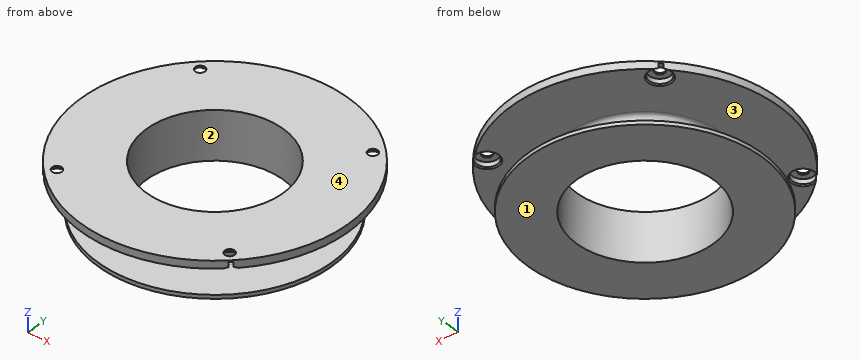
```python
from build123d import *

# Parameters (mm, degrees)
CBORE_FOR_10_BINDING_HEAD_MACHINE_S_2_COUNT = 2
CBORE_FOR_10_BINDING_HEAD_MACHINE_S_2_PITCH = 91.44
CBORE_FOR_10_BINDING_HEAD_MACHINE_S_3_COUNT = 2
CBORE_FOR_10_BINDING_HEAD_MACHINE_S_3_PITCH = 129.315688143
CBORE_FOR_10_BINDING_HEAD_MACHINE_S_4_COUNT = 2
CBORE_FOR_10_BINDING_HEAD_MACHINE_S_4_PITCH = 91.44


with BuildPart() as part:
    # Sketch1 → Revolve1 (revolve)
    with BuildSketch(Plane(origin=(0, 0, 0), x_dir=(1, 0, 0), z_dir=(0, 1, 0)), mode=Mode.PRIVATE) as revolve1_sk:
        with BuildLine():
            Line((-1.000000064, -24.96), (-1.000000064, -10.640000064))
            ThreePointArc((-1.000000064, -10.640000064), (-1.74394884, -8.84394884), (-3.540000064, -8.100000064))
            Line((-3.540000064, -8.100000064), (-24.4, -8.100000064))
            Line((-24.4, -8.100000064), (-24.4, -6.100000064))
            Line((-24.4, -6.100000064), (-1, -6.100000064))
            Line((-1, -6.100000064), (1, -6.100000064))
            Line((1, -6.100000064), (1, -31.500000128))
            Line((1, -31.500000128), (-33.29, -31.500000128))
            Line((-33.29, -31.500000128), (-33.29, -27.5))
            Line((-33.29, -27.5), (-3.540000064, -27.5))
            ThreePointArc((-3.540000064, -27.5), (-1.74394884, -26.756051224), (-1.000000064, -24.96))
        make_face()
    revolve(revolve1_sk.sketch.rotate(Axis((36.83, 0, 32.45), (0, 0, -1)), 180), axis=Axis((36.83, 0, 32.45), (0, 0, -1)))

    # Sketch7 → CBORE for #10 Binding Head Machine Screw1 (revolve, cut)
    with BuildSketch(Plane(origin=(82.55, 45.72, 27.5), x_dir=(0, 1, 0), z_dir=(1, 0, 0))):
        Polygon((0, 0), (0, 4.000000128), (2.5527, 4.000000128), (2.5527, 3.1242), (5.55625, 3.1242), (5.55625, 0.635), (6.19125, 0), align=None)
    cbore_for_10_binding_head_machine_screw = revolve(axis=Axis((82.55, 45.72, 21.15), (0, 0, 1)), mode=Mode.SUBTRACT)

    # CBORE for _10 Binding Head Machine S 2: CBORE for #10 Binding Head Machine Screw1 ×2
    with Locations(*[(-i * CBORE_FOR_10_BINDING_HEAD_MACHINE_S_2_PITCH, 0, 0) for i in range(1, CBORE_FOR_10_BINDING_HEAD_MACHINE_S_2_COUNT)]):
        add(cbore_for_10_binding_head_machine_screw, mode=Mode.SUBTRACT)

    # CBORE for _10 Binding Head Machine S 3: CBORE for #10 Binding Head Machine Screw1 ×2
    with Locations(*[Vector(-0.7071067811865476, -0.7071067811865476, 0) * (i * CBORE_FOR_10_BINDING_HEAD_MACHINE_S_3_PITCH) for i in range(1, CBORE_FOR_10_BINDING_HEAD_MACHINE_S_3_COUNT)]):
        add(cbore_for_10_binding_head_machine_screw, mode=Mode.SUBTRACT)

    # CBORE for _10 Binding Head Machine S 4: CBORE for #10 Binding Head Machine Screw1 ×2
    with Locations(*[(0, -i * CBORE_FOR_10_BINDING_HEAD_MACHINE_S_4_PITCH, 0) for i in range(1, CBORE_FOR_10_BINDING_HEAD_MACHINE_S_4_COUNT)]):
        add(cbore_for_10_binding_head_machine_screw, mode=Mode.SUBTRACT)


solid = part.part
```
Could you check a few things on this model? Use its own coordinates, in mm. Face numbers are marked on the shaded views. A direction names the side the tool comes from. Coordinates: 2 decimals unless noted, no trailing zeros. Write each loop counter-clockwise with the first axis right and the second up, starting at its lowest first coordinate (ties: lowest second). Pieces come first, ordered by that corner, then holes. Notation, with made-up numbers: (-8.5, 34.25) -> (49.5, 34.25) arc R30 ccw to (49.5, 60.25) -> close; hole circle Ø3 at (89, 45). An arc over 180 degrees is marked (long way). Return JSON: item names as keys, results as strings.
(1) Imagine slicing it at D-D, the plane z = 22. Please give me the cut outline in (x, y).
Numbers:
{"outline": "circle Ø75.66 at (36.83, 0); hole circle Ø71.66 at (36.83, 0)"}
(2) Imagine slicing it at A-A, the plane y = 0. Please give me the cut outline in (x, z).
Numbers:
{"outline": "(-33.29, 27.5) -> (-3.54, 27.5) arc R2.54 cw to (-1, 24.96) -> (-1, 10.64) arc R2.54 cw to (-3.54, 8.1) -> (-24.4, 8.1) -> (-24.4, 6.1) -> (1, 6.1) -> (1, 31.5) -> (-33.29, 31.5) -> close; (72.66, 6.1) -> (98.06, 6.1) -> (98.06, 8.1) -> (77.2, 8.1) arc R2.54 cw to (74.66, 10.64) -> (74.66, 24.96) arc R2.54 cw to (77.2, 27.5) -> (106.95, 27.5) -> (106.95, 31.5) -> (72.66, 31.5) -> close"}
(3) I'm going to push flat-ended pins straight in: pin 1 (1.5 mm diameter, centred on y = 12, z = 15, fed in from -X); pin 2 (4 mm diameter, centred on x = 38, z = 24.5, fed in from +Y); pin 3 (8 mm diameter, centred on x = 40, z = 13.5, fed in from -Y). Where does each tip first touch, or does it pass through?
Numbers:
{"pin 1": "stops at x = 0.71", "pin 2": "stops at y = 38.33", "pin 3": "stops at y = -37.99"}
(4) Imagine slicing it at B-B, the plane x = 36.83. Please give me the cut outline in (y, z), then the cut area to 3 significant figures.
Numbers:
{"outline": "(-70.12, 27.5) -> (-40.37, 27.5) arc R2.54 cw to (-37.83, 24.96) -> (-37.83, 10.64) arc R2.54 cw to (-40.37, 8.1) -> (-61.23, 8.1) -> (-61.23, 6.1) -> (-35.83, 6.1) -> (-35.83, 31.5) -> (-70.12, 31.5) -> close; (35.83, 6.1) -> (61.23, 6.1) -> (61.23, 8.1) -> (40.37, 8.1) arc R2.54 cw to (37.83, 10.64) -> (37.83, 24.96) arc R2.54 cw to (40.37, 27.5) -> (70.12, 27.5) -> (70.12, 31.5) -> (35.83, 31.5) -> close", "area": "459 mm2"}
(5) We'd pull the mould along Y, two halves only. Please class the marked faces 1 and 2: +Y half, -Y half, draft (parallel to the pull), parting line (faces both ways), or undercut.
Numbers:
{"face 1": "draft", "face 2": "undercut"}
(6) Which directions (+Z, -Z, +X, -X, +Y, -Y) give clear straight access to the entire face, cutting with the end or side of a thin tool? Please do the marked faces 3 and 4.
Numbers:
{"face 3": "none", "face 4": "+Z, +X, -X, +Y, -Y"}
(7) I need wall thicknesses on L1, parallel to Z at x = 96, y = 13; L2, parallel to Y at x = -8.89, z = 30; L3, parallel to X at y = 46, z = 29.75. Which ranges of each line are inside material? Lowest first, please.
Numbers:
{"L1": "z = 6.1 to 8.1, 27.5 to 31.5", "L2": "y = -53.16 to -51.28, -40.16 to 40.16, 51.28 to 53.16", "L3": "x = -16.09 to -14.44, -3.34 to 77, 88.1 to 89.75"}
(8) Imagine slicing it at C-C, the plane y = 45.72. Please give me the cut outline in (x, z) (3 decimals), then the cut area to 3 significant figures.
Numbers:
{"outline": "(-16.335, 27.5) -> (-15.081, 27.5) -> (-14.446, 28.135) -> (-14.446, 30.624) -> (-11.443, 30.624) -> (-11.443, 31.5) -> (-16.335, 31.5) -> close; (-6.337, 30.624) -> (-3.334, 30.624) -> (-3.334, 28.135) -> (-2.699, 27.5) -> (76.359, 27.5) -> (76.994, 28.135) -> (76.994, 30.624) -> (79.997, 30.624) -> (79.997, 31.5) -> (-6.337, 31.5) -> close; (-3.898, 6.1) -> (77.558, 6.1) -> (77.558, 8.1) -> (-3.898, 8.1) -> close; (85.103, 30.624) -> (88.106, 30.624) -> (88.106, 28.135) -> (88.741, 27.5) -> (89.995, 27.5) -> (89.995, 31.5) -> (85.103, 31.5) -> close", "area": "509 mm2"}
